from build123d import *

# Parameters (mm, degrees)
SCHIZZO1_W                   = 184
SCHIZZO1_H                   = 113
ESTRUSIONE_ESTRUSIONE1_DEPTH = 10
RACCORDO1_R                  = 2
RACCORDO2_R                  = 2
RACCORDO3_R                  = 2
RACCORDO4_R                  = 2
SCHIZZO2_W                   = 187
SCHIZZO2_H                   = 117
ESTRUSIONE_ESTRUSIONE2_DEPTH = 2.5
RACCORDO5_R                  = 3
RACCORDO6_R                  = 3
RACCORDO7_R                  = 3
RACCORDO8_R                  = 3


with BuildPart() as part:
    # Schizzo1 → Estrusione-Estrusione1 (new body)
    with BuildSketch(Plane.XY):
        Rectangle(SCHIZZO1_W, SCHIZZO1_H)
    extrude(amount=ESTRUSIONE_ESTRUSIONE1_DEPTH)

    # Raccordo1
    raccordo1_edges = [part.edges().sort_by_distance(p)[0] for p in [
        (-92, 56.5, 5),
    ]]
    fillet(raccordo1_edges, radius=RACCORDO1_R)

    # Raccordo2
    raccordo2_edges = [part.edges().sort_by_distance(p)[0] for p in [
        (-92, -56.5, 5),
    ]]
    fillet(raccordo2_edges, radius=RACCORDO2_R)

    # Raccordo3
    raccordo3_edges = [part.edges().sort_by_distance(p)[0] for p in [
        (92, -56.5, 5),
    ]]
    fillet(raccordo3_edges, radius=RACCORDO3_R)

    # Raccordo4
    raccordo4_edges = [part.edges().sort_by_distance(p)[0] for p in [
        (92, 56.5, 5),
    ]]
    fillet(raccordo4_edges, radius=RACCORDO4_R)

    # Schizzo2 → Estrusione-Estrusione2 (add)
    with BuildSketch(Plane.XY.offset(10)):
        Rectangle(SCHIZZO2_W, SCHIZZO2_H)
    extrude(amount=ESTRUSIONE_ESTRUSIONE2_DEPTH)

    # Raccordo5
    raccordo5_edges = [part.edges().sort_by_distance(p)[0] for p in [
        (-93.5, 58.5, 11.25),
    ]]
    fillet(raccordo5_edges, radius=RACCORDO5_R)

    # Raccordo6
    raccordo6_edges = [part.edges().sort_by_distance(p)[0] for p in [
        (-93.5, -58.5, 11.25),
    ]]
    fillet(raccordo6_edges, radius=RACCORDO6_R)

    # Raccordo7
    raccordo7_edges = [part.edges().sort_by_distance(p)[0] for p in [
        (93.5, -58.5, 11.25),
    ]]
    fillet(raccordo7_edges, radius=RACCORDO7_R)

    # Raccordo8
    raccordo8_edges = [part.edges().sort_by_distance(p)[0] for p in [
        (93.5, 58.5, 11.25),
    ]]
    fillet(raccordo8_edges, radius=RACCORDO8_R)


solid = part.part
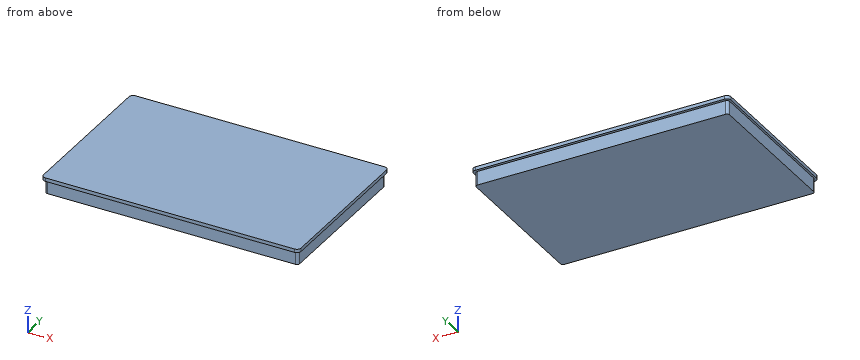
Here's how the part is built. I have some questions about the finished solid (model axes, mm). Coordinates: 2 decimals unless noted, no trailing zeros. Write each loop counter-clockwise with the first axis right and the second up, starting at its lowest first coordinate (ties: lowest second). Pieces come first, ordered by that corner, then holes.
1) If we section it at B-B (x = -52.5): List the corners of the cut face in (y, z) for me, plus the area to 3 significant figures.
Filled in:
outline: (-58.5, 10) - (-56.5, 10) - (-56.5, 0) - (56.5, 0) - (56.5, 10) - (58.5, 10) - (58.5, 12.5) - (-58.5, 12.5) - close
area: 1,420 mm2
2) If we section it at A-A (z = 4): List the corners of the cut face in (x, y) for me, plus the area to 3 significant figures.
Filled in:
outline: (-92, -54.5) arc R2 ccw to (-90, -56.5) - (90, -56.5) arc R2 ccw to (92, -54.5) - (92, 54.5) arc R2 ccw to (90, 56.5) - (-90, 56.5) arc R2 ccw to (-92, 54.5) - close
area: 20,800 mm2
3) If I drill on line 1 (Y direction, x = -52.5, z = 2); line 2 (X direction, y = -9, z = 8.25), over which ranges is the centre line in solid material (lowest first)?
Filled in:
line 1: y = -56.5 to 56.5
line 2: x = -92 to 92
4) I'm going to push flat-ended pins straight in: pin 1 (10 mm diameter, centred on x = 40.5, y = -19.5, fed in from -Z); pin 2 (6 mm diameter, centred on y = -31.5, z = 5.5, fed in from -X); pin 3 (5 mm diameter, centred on x = -11.5, z = 3.5, fed in from -Y); pin 4 (1.5 mm diameter, centred on y = 28, z = 5, fed in from +X). Where does each tip first touch, or does it pass through?
Filled in:
pin 1: stops at z = 0
pin 2: stops at x = -92
pin 3: stops at y = -56.5
pin 4: stops at x = 92
